Verification items for the finished model (mm, model axes). Face numbers are marked on the shaded views. A direction names the side the tool comes from. Give positions to 0.01 mm unless a question says otherwise; leave off trailing zeros. Loops run counter-clockwise (first coordinate to the right, second up) from the corner with the lowest first, then second, coordinate; pieces in that order, holes last. Notation, with made-up numbers: M -6.75,-11.75 L 35.25,-11.75 A19 ccw 35.25,24.25 Z; hole C -24.75,34 d8. An arc over 180 degrees is marked long. Answer in a Markdown table with one row per item.
Autodesk Fusion 360 part; units mm, degrees
sketch "Sketch1" plane through (0, 0, 0) normal (0, 0, 1) x (1, 0, 0)
  circle A0 centre (0, 0) radius 10.936
  dimension "d1" = 21.872
extrude "Extrude1" add sketch "Sketch1" along normal mid plane 18
sketch "Sketch2" plane through (0, 0, 9) normal (0, 0, 1) x (-1, 0, 0)
  circle A0 centre (0, 0) radius 10.936
  circle A1 centre (0, 0) radius 8.02
  dimension "d4" = 16.04
extrude "Extrude2" cut sketch "Sketch2" against normal blind 26 contours A1
sketch "Sketch3" plane through (0, 0, 0) normal (0, 1, 0) x (1, 0, 0)
  line L0 (-10.936, -9) -> (10.936, -9) construction
  line L1 (-10.936, 9) -> (10.936, 9) construction
  line L2 (10.936, -9) -> (10.936, 9) construction
  line L3 (10.936, 0) -> (9.936, 1.25)
  line L4 (9.936, 1.25) -> (10.936, 2.5)
  line L5 (10.936, 2.5) -> (10.936, 0)
  point P0 (10.936, 1.25)
  dimension "d7" = 2.5
  dimension "d8" = 1
revolve "Revolve1" cut sketch "Sketch3" angle 360 about axis through (0, 0, 1.75) along (0, 0, 1)
pattern_linear "R-Pattern1" count 4 spacing 2.5 along (0, 0, 1) both ways of "Revolve1"
ref_plane "WorkPlane1" through (0, 0, 2) normal (0, 0, -1) x (-1, 0, 0)
sketch "Sketch5" plane through (0, 0, 0) normal (0, 1, 0) x (1, 0, 0)
  line L0 (6.52, -2.5) -> (6.52, 2.5)
  line L1 (6.52, -2.5) -> (8.02, -4)
  line L2 (6.52, 2.5) -> (8.02, 4)
  line L3 (8.02, -4) -> (8.02, 4)
  point P0 (8.02, -9)
  point P1 (8.02, 9)
  point P2 (6.52, 0)
  dimension "d18" = 45
  dimension "d19" = 45
  dimension "d20" = 5
  dimension "d21" = 1.5
revolve "Revolve2" add sketch "Sketch5" angle 360 about axis through (0, 0, 1.75) along (0, 0, 1)
equation "d1 = 20.372 mm + 2 * teeth - 0.5 mm"
equation "d8 = teeth"
equation "teeth = 1 mm"
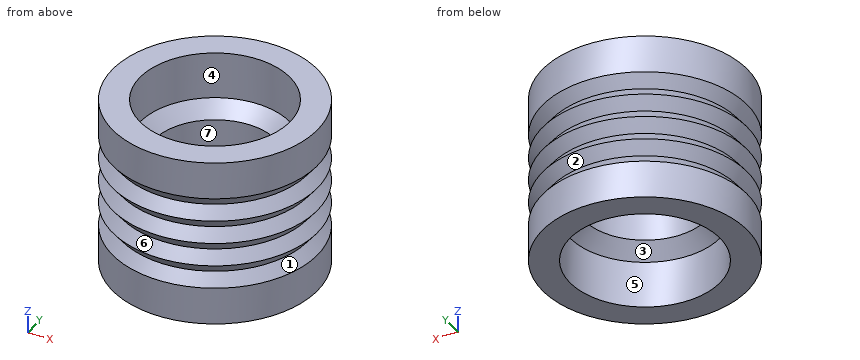
Item 1: Scan lines: L1, parallel to Z at x = -10, y = -3; L2, parallel to Y at x = 0, z = 7.8; L3, parallel to X at y = 0.5, z = -2.75. Record each from-to range of solid material in increasing order. Write a range as [from, to].
Reported:
| item | result |
|---|---|
| L1 | z = [-9, -4.38], [-3.12, -1.88], [-0.62, 0.62], [1.88, 3.12], [4.38, 9] |
| L2 | y = [-10.94, -8.02], [8.02, 10.94] |
| L3 | x = [-10.72, -6.75], [6.75, 10.72] |
Item 2: Release check for a two-part mould opening along Z. For the marked faces 1, 2, 3 and 4 record: released by +Z, released by -Z, zero draft, split by the parting line, or undercut.
Reported:
| item | result |
|---|---|
| face 1 | undercut |
| face 2 | undercut |
| face 3 | released by -Z |
| face 4 | zero draft |
Item 3: Go/stop test with flat-tipped pins: pin 1 (9.5 mm diameter, centred on x = 0, y = 0, fed in from +Z); pin 2 (1.5 mm diameter, centred on y = 5.5, z = -6, fed in from +X); pin 3 (3 mm diameter, centred on y = -4, z = -6, fed in from +X); pin 4 (2 mm diameter, centred on y = 2, z = 0, fed in from +X). Record where each tip stops, or that it passes through.
Reported:
| item | result |
|---|---|
| pin 1 | passes through |
| pin 2 | stops at x = 9.85 |
| pin 3 | stops at x = 10.65 |
| pin 4 | stops at x = 10.89 |
Item 4: Sectioned sample at C-C (z = -5.75). Record the cut outline in (x, y).
Reported:
| item | result |
|---|---|
| outline | C 0,0 d21.87; hole C 0,0 d16.04 |
Item 5: Tool access check on the marked faces 5, 6 and 7. Record the directions out of +Z, -Z, +X, -X, +Y, -Y that give a thin tool (end or side, any length) a straight path to the whole face; none if there is none.
Reported:
| item | result |
|---|---|
| face 5 | -Z |
| face 6 | none |
| face 7 | +Z, -Z |
